Autodesk Inventor part; units mm, degrees
ref_plane "YZ Plane" through (0, 0, 0) normal (1, 0, 0) x (0, 1, 0)
ref_plane "XZ Plane" through (0, 0, 0) normal (0, 1, 0) x (-1, 0, 0)
ref_plane "XY Plane" through (0, 0, 0) normal (0, 0, 1) x (1, 0, 0)
sketch "Sketch1" plane through (0, 0, 0) normal (1, 0, 0) x (0, 1, 0)
  circle A0 centre (0, 0) radius 1.5
  arc A1 (3.5, 0) -> (0, -3.5) centre (0, 0) ccw
  line L0 (0, 0) -> (0, -18)
  circle A2 centre (0, -18) radius 1.5
  line L1 (0, -18) -> (0, -28)
  circle A3 centre (0, -28) radius 1.5
  arc A4 (0, -24.5) -> (3.5, -28) centre (0, -28) ccw
  line L2 (3.5, 0) -> (3.5, -28)
  line L3 (-3.5, 0) -> (-3.5, -28)
  dimension "d0" = 3
  dimension "d1" = 7
  dimension "d2" = 18
  dimension "d3" = 3
  dimension "d4" = 10
  dimension "d5" = 3
  dimension "d6" = 7
extrude "Extrusion1" add sketch "Sketch1" along normal blind 3 contours A1 L2 A4 L1 A2 L0 | L0 A2 L1 A4 L3 A1
properties part number "acople_gripper"
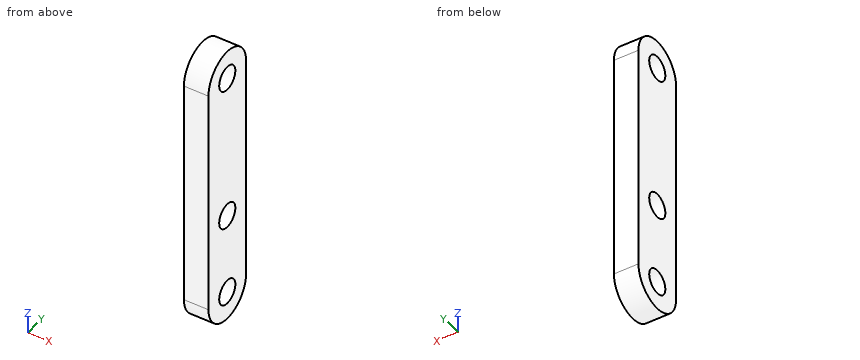
Check sheet for the modelled part. Datum: model origin and axes. Units: mm. Round coordinates to 2 decimals unless told otherwise and drop trailing zeros. Loops run counter-clockwise (first coordinate to the right, second up) from the corner with the lowest first, then second, coordinate; pieces in that order, holes last. Notation, with made-up numbers: M -10.5,49.5 L 1.5,49.5 A20 ccw 1.5,85.5 Z; hole C -7.5,-30.75 d5. An arc over 180 degrees is marked long. Answer as a JSON object with one key per item and string values.
1. Section check D-D (y = -2.75). Record the boundary of the cut face in (x, z).
Reply:
{"outline": "M 0,-30.17 L 3,-30.17 L 3,2.17 L 0,2.17 Z"}
2. Section check A-A (y = 0). Record the boundary of the cut face in (x, z).
Reply:
{"outline": "M 0,-31.5 L 3,-31.5 L 3,-29.5 L 0,-29.5 Z; M 0,-26.5 L 3,-26.5 L 3,-19.5 L 0,-19.5 Z; M 0,-16.5 L 3,-16.5 L 3,-1.5 L 0,-1.5 Z; M 0,1.5 L 3,1.5 L 3,3.5 L 0,3.5 Z"}
3. Section check C-C (y = 2.25). Record the boundary of the cut face in (x, z), plus the area to 3 significant figures.
Reply:
{"outline": "M 0,-30.68 L 3,-30.68 L 3,2.68 L 0,2.68 Z", "area": "100 mm²"}
4. Scan lines: line 1 (Z direction, x = 0.95, y = 0); line 2 (Y direction, x = 2.2, z = 0); line 3 (Z direction, x = 0.8, y = -0.75). Record each from-to range of solid material in increasing order.
Reply:
{"line 1": "z = -31.5 to -29.5, -26.5 to -19.5, -16.5 to -1.5, 1.5 to 3.5", "line 2": "y = -3.5 to -1.5, 1.5 to 3.5", "line 3": "z = -31.42 to -29.3, -26.7 to -19.3, -16.7 to -1.3, 1.3 to 3.42"}
5. Gauge pin test, flat ends, axial feed: P1, Ø3.5, axis at y = 0, z = 0, coming from the +X side; P2, Ø1.5, axis at x = 1.5, y = -1, coming from the -Z side. Record the tip position at first contact, or that the pin passes through.
Reply:
{"P1": "stops at x = 3", "P2": "stops at z = -31.49"}
6. Section check B-B (x = 2.45). Record the boundary of the cut face in (y, z).
Reply:
{"outline": "M -3.5,-28 A3.5 ccw 3.5,-28 L 3.5,0 A3.5 ccw -3.5,0 Z; hole C 0,-28 d3; hole C 0,-18 d3; hole C 0,0 d3"}
